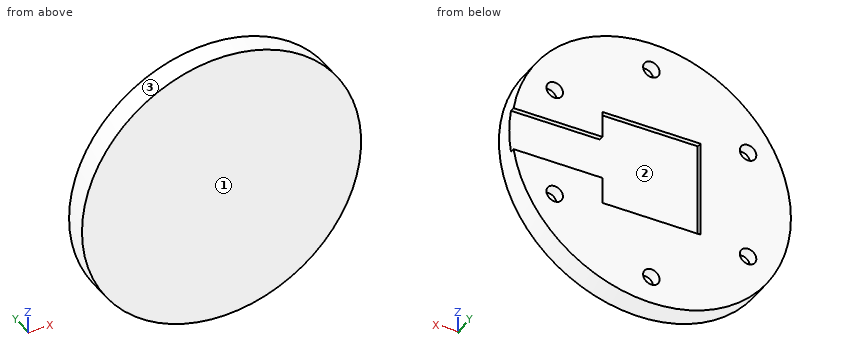
Autodesk Inventor part; units mm, degrees
ref_plane "YZ Plane" through (0, 0, 0) normal (1, 0, 0) x (0, 1, 0)
ref_plane "XZ Plane" through (0, 0, 0) normal (0, 1, 0) x (-1, 0, 0)
ref_plane "XY Plane" through (0, 0, 0) normal (0, 0, 1) x (1, 0, 0)
sketch "Szkic1" plane through (0, 0, 0) normal (0, 1, 0) x (-1, 0, 0)
  circle A0 centre (0, 0) radius 60
  dimension "d0" = 120
extrude "Wyciągnięcie proste1" add sketch "Szkic1" along normal blind 10
sketch "Szkic2" plane through (0, 10, 0) normal (0, 1, 0) x (1, 0, 0)
  circle A0 centre (0, 48) radius 3.55
  circle A1 centre (-41.5692, 24) radius 3.55
  circle A2 centre (-41.5692, -24) radius 3.55
  circle A3 centre (0, -48) radius 3.55
  circle A4 centre (41.5692, -24) radius 3.55
  circle A5 centre (41.5692, 24) radius 3.55
  point P0 (0, 0)
  dimension "d13" = 7.1
  dimension "d16" = 360
  dimension "d20" = 48
extrude "Wyciągnięcie proste2" cut sketch "Szkic2" against normal blind 5
sketch "Szkic3" plane through (0, 10, 0) normal (0, 1, 0) x (1, 0, 0)
  line L0 (-21.05, -21.05) -> (21.05, -21.05)
  line L1 (21.05, -21.05) -> (21.05, 21.05)
  line L2 (21.05, 21.05) -> (-21.05, 21.05)
  line L3 (-21.05, 21.05) -> (-21.05, -21.05)
  line L4 (-21.05, -21.05) -> (21.05, 21.05)
  line L5 (-21.05, 21.05) -> (21.05, -21.05)
  point P0 (0, 0)
  point P1 (0, 0)
  dimension "d21" = 42.1
  dimension "d22" = 42.1
extrude "Wyciągnięcie proste3" cut sketch "Szkic3" against normal blind 2
sketch "Szkic4" plane through (0, 10, 0) normal (0, 1, 0) x (1, 0, 0)
  line L0 (21.05, 21.05) -> (21.05, -21.05)
  line L1 (21.05, -9.5) -> (61.05, -9.5)
  line L2 (61.05, -9.5) -> (61.05, 9.5)
  line L3 (61.05, 9.5) -> (21.05, 9.5)
  line L4 (21.05, 9.5) -> (21.05, -9.5)
  point P0 (0, 0)
  point P1 (21.05, 0)
  dimension "d25" = 19
  dimension "d26" = 40
extrude "Wyciągnięcie proste4" cut sketch "Szkic4" against normal blind 2
properties part number "Base1"
Can you work these out from the model? Positions are in its coordinate system, mm. Face numbers are marked on the shaded views. Coordinates: 2 decimals unless noted, no trailing zeros. Write each loop counter-clockwise with the first axis right and the second up, starting at its lowest first coordinate (ties: lowest second). Pieces come first, ordered by that corner, then holes. Notation, with made-up numbers: M -3,-22 L 33,-22 A17 cw 33,-5 Z; hole C 25,66.5 d2. An arc over 180 degrees is marked long. Answer as CSV lines item,"result".
Item 1: Please list where these lines run through material, in increasing order: line 1 along Z through (x, y) = (0, 8.85); line 2 along X through (y, z) = (6.15, -24); line 3 along Z through (x, y) = (-3, 5.25).
Geometry results:
line 1,"z = -60 to -51.55, -44.45 to -21.05, 21.05 to 44.45, 51.55 to 60"
line 2,"x = -54.99 to -45.12, -38.02 to 38.02, 45.12 to 54.99"
line 3,"z = -59.92 to -49.9, -46.1 to 46.1, 49.9 to 59.92"
Item 2: We'd pull the mould along X, two halves only. Please class the marked faces 1, 2 and 3: +X half, -X half, draft (parallel to the pull), parting line (faces both ways), or undercut.
Geometry results:
face 1,"draft"
face 2,"undercut"
face 3,"parting line"
Item 3: Imagine slicing it at A-A on z = -48. List the corners of the cut face in (x, y) for me, plus the area to 4 significant figures.
Geometry results:
outline,"M -36,0 L 36,0 L 36,10 L 3.55,10 L 3.55,5 L -3.55,5 L -3.55,10 L -36,10 Z"
area,"684.5 mm2"
Item 4: Imagine slicing it at D-D on z = 24. List the corners of the cut face in (x, y) for me.
Geometry results:
outline,"M -54.99,0 L 54.99,0 L 54.99,10 L 45.12,10 L 45.12,5 L 38.02,5 L 38.02,10 L -38.02,10 L -38.02,5 L -45.12,5 L -45.12,10 L -54.99,10 Z"
Item 5: Imagine slicing it at C-C on y = 1.5. List the corners of the cut face in (x, z) for me.
Geometry results:
outline,"C 0,0 d120"
Item 6: Imagine slicing it at B-B on x = 27.5. List the corners of the cut face in (y, z) for me, plus the area to 3 significant figures.
Geometry results:
outline,"M 0,-53.33 L 10,-53.33 L 10,-9.5 L 8,-9.5 L 8,9.5 L 10,9.5 L 10,53.33 L 0,53.33 Z"
area,"1,030 mm2"
Item 7: I'm going to push flat-ended pins straight in: P1, Ø6, axis at x = 14, y = 2, coming from the -Z side; P2, Ø1.6, axis at y = 9, z = 2, coming from the +X side; P3, Ø2, axis at y = 8.5, z = -15, coming from the -X side. Where does each tip first touch, or does it pass through?
Geometry results:
P1,"stops at z = -58.98"
P2,"stops at x = -21.05"
P3,"stops at x = -58.34"
